Check sheet for the drawn part. Datum: minimum x, y, z corner. Units: mm. A direction names the side the tool comes from. Round coordinates to 2 decimals unless told otherwise and drop trailing zeros. Write each loop counter-clockwise with the first axis right and the second up, starting at its lowest first coordinate (ties: lowest second). Pieces come first, ordered by that corner, then holes. Notation, with made-up numbers: M 9,50.5 L 19,50.5 A26 ccw 19,85.5 Z; hole C -21,-31 d8. An arc over 180 degrees is marked long. One line per item, written item: value. Start each with the question number.
Item 1: Section check D-D, the plane z = 85.5. Record the cut outline in (x, y).
Item 2: Thickness scan on probe 1 along Y at (x, z) = (13.5, 69); probe 2 along Z at (x, y) = (22.5, 95.25); probe 3 along X at (y, z) = (11, 22) (1 decimal). Record the ranges inside material, lowest first. Write a range as from..to.
Item 3: Draft check along Z on the marked faces 4, 5, 6 and 7. Enter one of: +Z half, -Z half, draft (parallel to the pull), parting line (faces both ways), or undercut.
Item 4: Section check C-C, the plane y = 93.5. Record the cut outline in (x, z), then the cut area to 3 significant figures.
Item 5: Tool access check on the marked faces 1, 2 and 3. Record the directions out of +Z, -Z, +X, -X, +Y, -Y that give a thin tool (end or side, any length) a straight path to the whole face; none if there is none.
Item 6: Section check A-A, the plane x = 22.5. Record the cut outline in (y, z).
Item 7: Section check B-B, the plane z = 17.5. Record the cut outline in (x, y).
Item 8: Gauge pin test, flat ends, axial feed: pin 1 (10 mm diameter, centred on x = 38.5, y = 59.5, fed in from -Z); pin 2 (6 mm diameter, centred on y = 13.5, z = 27, fed in from +X). Record the tip position at first contact, or that the pin passes through.
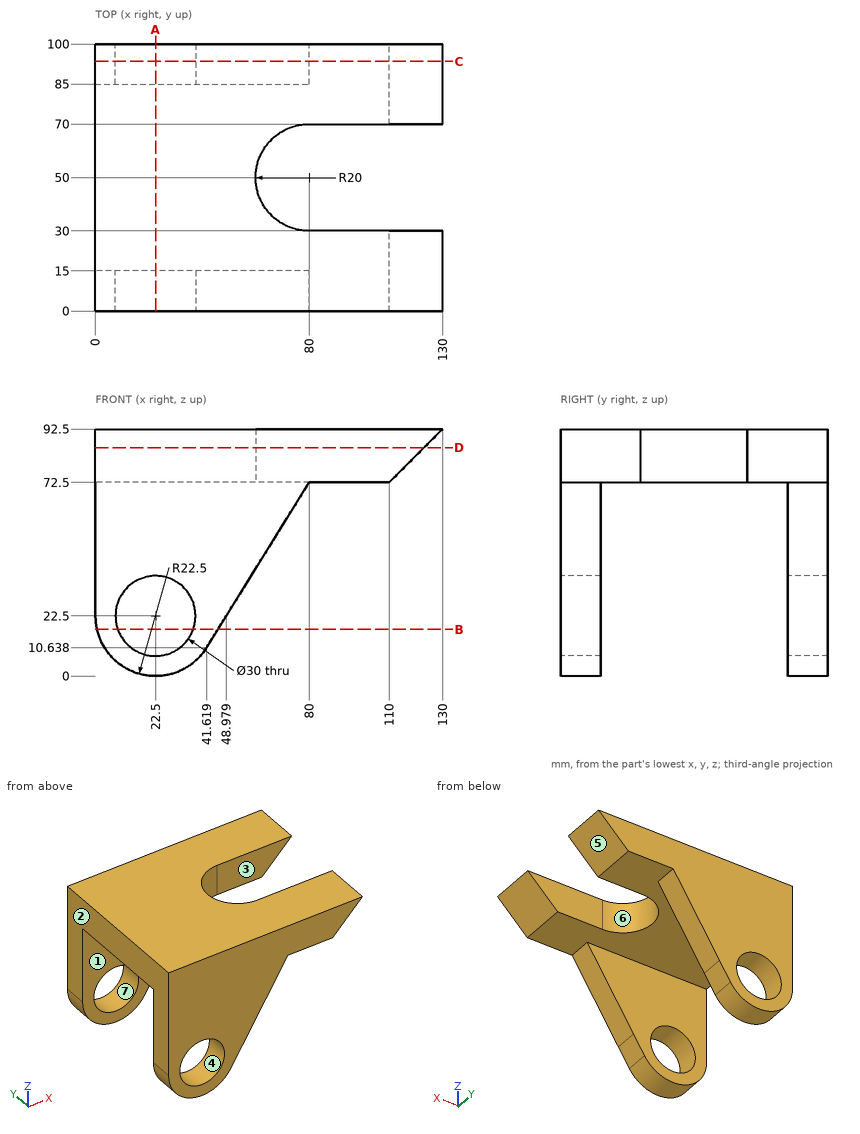
Response values:
1. outline: M 0,0 L 123,0 L 123,30 L 80,30 A20 cw 80,70 L 123,70 L 123,100 L 0,100 Z
2. probe 1: y = 0..15, 85..100
2. probe 2: z = 0..7.5, 37.5..92.5
2. probe 3: x = 0..7.5, 37.5..48.7
3. face 4: undercut
3. face 5: -Z half
3. face 6: draft
3. face 7: undercut
4. outline: M 0,22.5 A22.5 ccw 41.62,10.64 L 80,72.5 L 110,72.5 L 130,92.5 L 0,92.5 Z; hole C 22.5,22.5 d30
4. area: 5,730 mm2
5. face 1: -Z, +X, -X
5. face 2: +Z, -Z, -X, +Y, -Y
5. face 3: +Z, -Z, +X
6. outline: M 0,0 L 15,0 L 15,7.5 L 0,7.5 Z; M 0,37.5 L 15,37.5 L 15,72.5 L 85,72.5 L 85,37.5 L 100,37.5 L 100,92.5 L 0,92.5 Z; M 85,0 L 100,0 L 100,7.5 L 85,7.5 Z
7. outline: M 0.56,0 L 8.36,0 L 8.36,15 L 0.56,15 Z; M 0.56,85 L 8.36,85 L 8.36,100 L 0.56,100 Z; M 36.64,0 L 45.88,0 L 45.88,15 L 36.64,15 Z; M 36.64,85 L 45.88,85 L 45.88,100 L 36.64,100 Z
8. pin 1: stops at z = 72.5
8. pin 2: stops at x = 53.63
